Verification items for the finished model (mm, model axes). Round coordinates to 2 decimals unless told otherwise and drop trailing zeros. Write each loop counter-clockwise with the first axis right and the second up, starting at its lowest first coordinate (ties: lowest second). Pieces come first, ordered by that corner, then holes. Notation, with made-up numbers: M 39.5,79 L 55.5,79 A17 cw 55.5,84 Z; hole C -7,19.25 d2. An arc over 180 degrees is marked long. One line per question, with ' | ' between items.
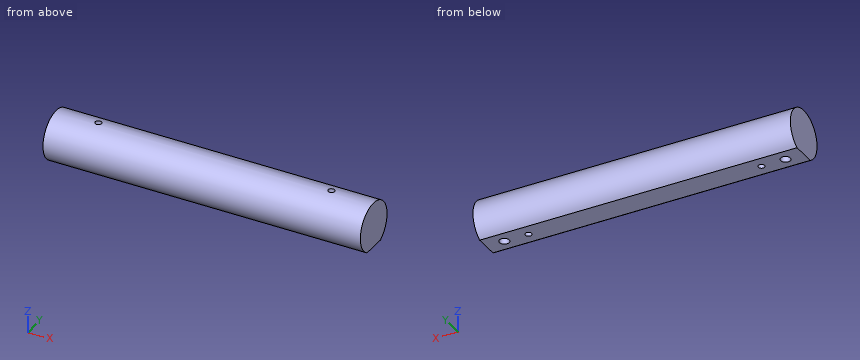
from build123d import *

# Parameters (mm, degrees)
F1_DEPTH = 395
F2_R     = 6
F2_R_2   = 4
F3_DEPTH = 43
F4_R     = 4
F5_DEPTH = 71
F6_SIZE  = 6


with BuildPart() as f1:
    # F0 (on Right) → F1 (new body)
    with BuildSketch(Plane.YZ):
        with BuildLine():
            Line((-14.96663, -26), (14.96663, -26))
            ThreePointArc((14.96663, -26), (0, 30), (-14.96663, -26))
        make_face()
    extrude(amount=F1_DEPTH)

    # F2 (on face) → F3 (cut)
    with BuildSketch(Plane(origin=(0, 0, -26), x_dir=(1, 0, 0), z_dir=(0, 0, -1))):
        with Locations((372.5, 0)):
            Circle(F2_R)
        with Locations((22.5, 0)):
            Circle(F2_R)
        with Locations((52.5, 0)):
            Circle(F2_R_2)
        with Locations((342.5, 0)):
            Circle(F2_R_2)
    extrude(amount=-F3_DEPTH, mode=Mode.SUBTRACT)

    # F4 (on face) → F5 (cut)
    with BuildSketch(Plane(origin=(0, 0, -26), x_dir=(1, 0, 0), z_dir=(0, 0, -1))):
        with Locations((52.5, 0)):
            Circle(F4_R)
        with Locations((342.5, 0)):
            Circle(F4_R)
    extrude(amount=-F5_DEPTH, mode=Mode.SUBTRACT)

    # F6
    f6_edges = [f1.edges().sort_by_distance(p)[0] for p in [
        (366.5, 0, 17),
        (16.5, 0, 17),
    ]]
    chamfer(f6_edges, length=F6_SIZE)


solid = f1.part
1. Section check A-A, the plane z = -17. Record the cut outline in (x, y).
Results:
outline: M 0,-24.72 L 395,-24.72 L 395,24.72 L 0,24.72 Z; hole C 22.5,0 d12; hole C 52.5,0 d8; hole C 342.5,0 d8; hole C 372.5,0 d12
2. Section check B-B, the plane x = 52.5. Record the cut outline in (y, z).
Results:
outline: M -14.97,-26 L -4,-26 L -4,29.73 A30 ccw Z; M 4,-26 L 14.97,-26 A30 ccw 4,29.73 Z
3. Thickness scan on line 1 (X direction, y = 0, z = -9); line 2 (Y direction, x = 52, z = -1); line 3 (Y direction, x = 52.5, z = 2). Record the ranges inside material, lowest first.
Results:
line 1: x = 0 to 16.5, 28.5 to 48.5, 56.5 to 338.5, 346.5 to 366.5, 378.5 to 395 | line 2: y = -29.98 to -3.97, 3.97 to 29.98 | line 3: y = -29.93 to -4, 4 to 29.93
4. Go/stop test with flat-tipped pins: P1, Ø4, axis at x = 168, z = 23.5, coming from the -Y side; P2, Ø8, axis at x = 334, z = -8, coming from the -Y side; P3, Ø4, axis at x = 41, y = -6.5, coming from the +Z side. Record where each tip stops, or that it passes through.
Results:
P1: stops at y = -20.92 | P2: stops at y = -29.73 | P3: stops at z = 29.66
5. Section check D-D, the plane y = -23.5. Record the cut outline in (x, z), then the cut area to 3 significant figures.
Results:
outline: M 0,-18.65 L 395,-18.65 L 395,18.65 L 0,18.65 Z | area: 14,700 mm2
6. Section check C-C, the plane x = 253. Record the cut outline in (y, z).
Results:
outline: M -14.97,-26 L 14.97,-26 A30 ccw long Z
